Source: CAD feature listing. Evaluate the final solid. Frame: model axes, mm. Face numbers are marked on the shaded views. Coordinates: 2 decimals unless noted, no trailing zeros. Loops run counter-clockwise (first coordinate to the right, second up) from the corner with the lowest first, then second, coordinate; pieces in that order, holes last.
from build123d import *

# Parameters (mm, degrees)
SKETCH1_R           = 6.35
SKETCH1_R_2         = 0.762
BOSS_EXTRUDE1_DEPTH = 3.175


with BuildPart() as part:
    # Sketch1 → Boss-Extrude1 (new body)
    with BuildSketch(Plane.XY):
        Circle(SKETCH1_R)
        with Locations((0, 4.7625)):
            Circle(SKETCH1_R_2, mode=Mode.SUBTRACT)
        with Locations((4.7625, 0)):
            Circle(SKETCH1_R_2, mode=Mode.SUBTRACT)
        with Locations((0, -4.7625)):
            Circle(SKETCH1_R_2, mode=Mode.SUBTRACT)
        with Locations((-4.7625, 0)):
            Circle(SKETCH1_R_2, mode=Mode.SUBTRACT)
        with BuildLine():
            Line((-1.782587852, -2.35077), (1.782587852, -2.35077))
            ThreePointArc((1.782587852, -2.35077), (0, 2.95021), (-1.782587852, -2.35077))
        make_face(mode=Mode.SUBTRACT)
    extrude(amount=BOSS_EXTRUDE1_DEPTH)


solid = part.part
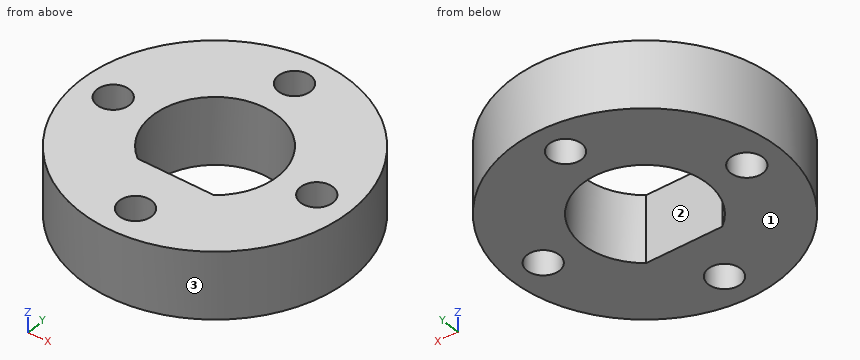
Q1. Section D-D, the plane y = -0.5. Return the cut outline in (x, z) (3 decimals), plus the area to 3 significant figures.
Q2. Line query: line 1 along Y through (x, z) = (0, 0.8); line 2 along Y through (x, z) = (-0.5, 0.9); line 3 along X through (y, z) = (-1.75, 0.6). Output: solid intervals per line, ascending.
Q3. Section B-B, the plane y = 1. Return the cut outline in (x, z) (3 decimals).
Q4. Section A-A, the plane x = 0. Count the separate pieces of the cut face and the enclosed holes in it, plus the area to 3 significant figures.
Q5. Section C-C, the plane x = 4.75. Return the cut outline in (y, z) (3 decimals).
Q6. Contact query for flat-ended pins moving along their axis: pin 1 Ø6 at (x, y) = (4.5, 0.5) entering from -Z; pin 2 Ø0.9 at (x, y) = (0, 4.76) entering from +Z; pin 3 Ø1 at (x, z) = (1, 2) entering from +Y. Output: stop coordinate, or through.
Q7. Draft query along X for the marked faces 1, 2 and 3. Return one class per face: +X half, -X half, draft (parallel to the pull), parting line (faces both ways), or undercut.
Derived:
1. outline: (-6.33, 0) - (-5.338, 0) - (-5.338, 3.175) - (-6.33, 3.175) - close; (-4.187, 0) - (-2.908, 0) - (-2.908, 3.175) - (-4.187, 3.175) - close; (2.908, 0) - (4.187, 0) - (4.187, 3.175) - (2.908, 3.175) - close; (5.338, 0) - (6.33, 0) - (6.33, 3.175) - (5.338, 3.175) - close
1. area: 14.4 mm2
2. line 1: y = -6.35 to -5.52, -4 to -2.35, 2.95 to 4, 5.52 to 6.35
2. line 2: y = -6.33 to -5.34, -4.19 to -2.35, 2.91 to 4.19, 5.34 to 6.33
2. line 3: x = -6.1 to -2.38, 2.38 to 6.1
3. outline: (-6.271, 0) - (-2.776, 0) - (-2.776, 3.175) - (-6.271, 3.175) - close; (2.776, 0) - (6.271, 0) - (6.271, 3.175) - (2.776, 3.175) - close
4. separate pieces: 4
4. enclosed holes: 0
4. area: 13.8 mm2
5. outline: (-4.214, 0) - (-0.762, 0) - (-0.762, 3.175) - (-4.214, 3.175) - close; (0.762, 0) - (4.214, 0) - (4.214, 3.175) - (0.762, 3.175) - close
6. pin 1: stops at z = 0
6. pin 2: passes through
6. pin 3: stops at y = 6.33
7. face 1: draft
7. face 2: undercut
7. face 3: parting line
